from build123d import *

# Parameters (mm, degrees)
BODYSKETCH_W              = 165
BODYSKETCH_H              = 50
BODY_DEPTH                = 38
HOLESKETCH_W              = 34
HOLESKETCH_H              = 46
HOLE_DEPTH                = 163
SECONDBATTERYSKETCH_W     = 87
SECONDBATTERYSKETCH_H     = 44
SECONDBATTERY_DEPTH       = 39
SECONDBATTERYHOLESKETCH_W = 37
SECONDBATTERYHOLESKETCH_H = 40
SECONDBATTERYHOLE_DEPTH   = 85
CONNECTORSKETCH_R         = 2
CUT_EXTRUDE3_DEPTH        = 15
STRAPSKETCH_W             = 20
STRAPSKETCH_H             = 3
CUT_EXTRUDE4_DEPTH        = 51
CUT_EXTRUDE5_DEPTH        = 51
CUT_EXTRUDE6_DEPTH        = 166


with BuildPart() as part:
    # BodySketch → Body (new body)
    with BuildSketch(Plane(origin=(0, 0, 0), x_dir=(0, 0, -1), z_dir=(1, 0, 0))):
        Rectangle(BODYSKETCH_W, BODYSKETCH_H)
    extrude(amount=BODY_DEPTH)

    # HoleSketch → Hole (cut)
    with BuildSketch(Plane.XY.offset(82.5)):
        with Locations((19, 0)):
            Rectangle(HOLESKETCH_W, HOLESKETCH_H)
    extrude(amount=-HOLE_DEPTH, mode=Mode.SUBTRACT)

    # SecondBatterySketch → SecondBattery (add)
    with BuildSketch(Plane.ZY):
        Rectangle(SECONDBATTERYSKETCH_W, SECONDBATTERYSKETCH_H)
    extrude(amount=SECONDBATTERY_DEPTH)

    # SecondBatteryHoleSketch → SecondBatteryHole (cut)
    with BuildSketch(Plane.XY.offset(43.5)):
        with Locations((-18.5, 0)):
            Rectangle(SECONDBATTERYHOLESKETCH_W, SECONDBATTERYHOLESKETCH_H)
    extrude(amount=-SECONDBATTERYHOLE_DEPTH, mode=Mode.SUBTRACT)

    # ConnectorSketch → Cut-Extrude3 (cut)
    with BuildSketch(Plane(origin=(38, 0, 0), x_dir=(0, 0, -1), z_dir=(1, 0, 0))):
        with Locations((-70, 17)):
            Circle(CONNECTORSKETCH_R)
        with Locations((-70, -17)):
            Circle(CONNECTORSKETCH_R)
        with Locations((70, -17)):
            Circle(CONNECTORSKETCH_R)
    extrude(amount=-CUT_EXTRUDE3_DEPTH, mode=Mode.SUBTRACT)

    # StrapSketch → Cut-Extrude4 (cut, through all)
    with BuildSketch(Plane(origin=(0, 25, 0), x_dir=(1, 0, 0), z_dir=(0, 1, 0))):
        with Locations((19, -77.5)):
            Rectangle(STRAPSKETCH_W, STRAPSKETCH_H)
        with Locations((-19.5, -38.5)):
            Rectangle(STRAPSKETCH_W, STRAPSKETCH_H)
    extrude(amount=-CUT_EXTRUDE4_DEPTH, mode=Mode.SUBTRACT)

    # WeightReduction → Cut-Extrude5 (cut, through all)
    with BuildSketch(Plane(origin=(0, 25, 0), x_dir=(1, 0, 0), z_dir=(0, 1, 0))):
        Polygon((4.8, 77.5), (4.8, 44.7), (33.205633244, 61.1), align=None)
        Polygon((33.205633244, -19.5), (33.205633244, -52.3), (4.8, -35.9), align=None)
        Polygon((33.205633244, 58.1), (33.205633244, 25.3), (4.8, 41.7), align=None)
        Polygon((4.8, 38.7), (4.8, 5.9), (33.205633244, 22.3), align=None)
        Polygon((33.205633244, 19.3), (33.205633244, -13.5), (4.8, 2.9), align=None)
        Polygon((4.8, -0.1), (4.8, -32.9), (33.205633244, -16.5), align=None)
        Polygon((4.8, -38.9), (4.8, -71.7), (33.205633244, -55.3), align=None)
        Polygon((33.205633244, -58.3), (33.205633244, -71.7), (9.996152423, -71.7), align=None)
        Polygon((33.205633244, 64.1), (33.205633244, 77.5), (9.996152423, 77.5), align=None)
        Polygon((-34.2, 38.5), (-34.2, 10.5), (-9.951288694, 24.5), align=None)
        Polygon((-9.951288694, 21.5), (-9.951288694, -6.5), (-34.2, 7.5), align=None)
        Polygon((-34.2, 4.5), (-34.2, -23.5), (-9.951288694, -9.5), align=None)
        Polygon((-34.2, -26.5), (-9.951288694, -12.5), (-9.951288694, -34), (-21.209618943, -34), align=None)
        Polygon((-9.951288694, 27.5), (-9.951288694, 39.047005384), (-29.951288694, 39.047005384), align=None)
    extrude(amount=-CUT_EXTRUDE5_DEPTH, mode=Mode.SUBTRACT)

    # weightCut → Cut-Extrude6 (cut, through all)
    with BuildSketch(Plane(origin=(0, 0, -82.5), x_dir=(-1, 0, 0), z_dir=(0, 0, -1))):
        Polygon((-31, -20), (-19, -2.862223919), (-7, -20), align=None)
        Polygon((-33, -18), (-20.396264312, 0), (-33, 18), align=None)
        Polygon((-31, 20), (-19, 2.862223919), (-7, 20), align=None)
        Polygon((-5, 18), (-17.603735688, 0), (-5, -18), align=None)
        Polygon((8, -19), (19.5, -2.576297922), (31, -19), align=None)
        Polygon((6, -17), (17.90352815, 0), (6, 17), align=None)
        Polygon((33, -17), (21.09647185, 0), (33, 17), align=None)
        Polygon((8, 19), (19.5, 2.576297922), (31, 19), align=None)
    extrude(amount=-CUT_EXTRUDE6_DEPTH, mode=Mode.SUBTRACT)


solid = part.part
The listing builds one solid part. Answer for the finished solid, in the listing's coordinates (mm). A direction names the side the tool comes from. Coordinates: 2 decimals unless noted, no trailing zeros. Write each loop counter-clockwise with the first axis right and the second up, starting at its lowest first coordinate (ties: lowest second). Pieces come first, ordered by that corner, then holes. Notation, with made-up numbers: (21.25, 39.25) - (56.25, 39.25) arc R37 cw to (56.25, 75.25) - close; hole circle Ø1 at (81, 72.5). An arc over 180 degrees is marked (long way). Answer as CSV lines item,"result".
1. Find section A-A (z = -70). Give the vertices of the cut face in (x, y).
Computed values:
outline,"(0, -25) - (4.8, -25) - (4.8, -23) - (2, -23) - (2, 23) - (4.8, 23) - (4.8, 25) - (0, 25) - close; (17.79, -25) - (22.99, -25) - (22.99, -23) - (17.79, -23) - close; (17.79, 23) - (22.99, 23) - (22.99, 25) - (17.79, 25) - close; (33.21, -25) - (38, -25) - (38, -19) - (36, -19) - (36, -23) - (33.21, -23) - close; (33.21, 23) - (36, 23) - (36, -15) - (38, -15) - (38, 25) - (33.21, 25) - close"
2. Find section B-B (z = 70). Give the number of separate pieces and of enclosed holes in the cut face, plus the area to 3 significant figures.
Computed values:
separate pieces,"6"
enclosed holes,"0"
area,"227 mm²"
3. Straight lines are drawn through the part: line 1 (X direction, y = -18.5, z = 15); line 2 (Y direction, x = 37.55, z = 70); line 3 (X direction, y = -21, z = 53.5). For each, find the intervals that lie inside material, in ascending order. Write a range as [from, to].
Computed values:
line 1,"x = [-39, -37], [0, 2], [36, 38]"
line 2,"y = [-25, -19], [-15, 15], [19, 25]"
line 3,"x = [0, 2], [36, 38]"
4. Given P1, Ø2.5, axis at y = -17, z = -70, coming from the -X side; P2, Ø0.6, axis at x = -13.5, y = 20.5, coming from the -Z side; P3, Ø10, axis at x = -28.5, y = 19, coming from the +Z side, each flat-ended and moving along its own axis, determine where each tip first touches the part or whether it passes through.
Computed values:
P1,"stops at x = 0"
P2,"stops at z = -43.5"
P3,"stops at z = 43.5"
5. Determine the mould class of faces 1 (the cylindrical face through (37.014, -15.314, 68.925)), 2 (the flat face through (-39, 0, -1)), 3 (the flat face through (-37, 0, 2)) for opening direction X: +X half, -X half, draft (parallel to the pull), parting line (faces both ways), or undercut.
Computed values:
face 1,"draft"
face 2,"-X half"
face 3,"undercut"
6. A tool of negligible diameter and unlimited length cuts with its end or side. For faces 4 (the flat face through (-20.091, 21.014, -33.354)), 5 (the flat face through (2, 0, 2)), 6 (the flat face through (-13.67, -10.9, -42.51)), from which of +Z, -Z, +X, -X, +Y, -Y can it reach the whole face along a straight path? Write none if from no direction.
Computed values:
face 4,"+Y, -Y"
face 5,"+Z"
face 6,"+Z, -Z"
